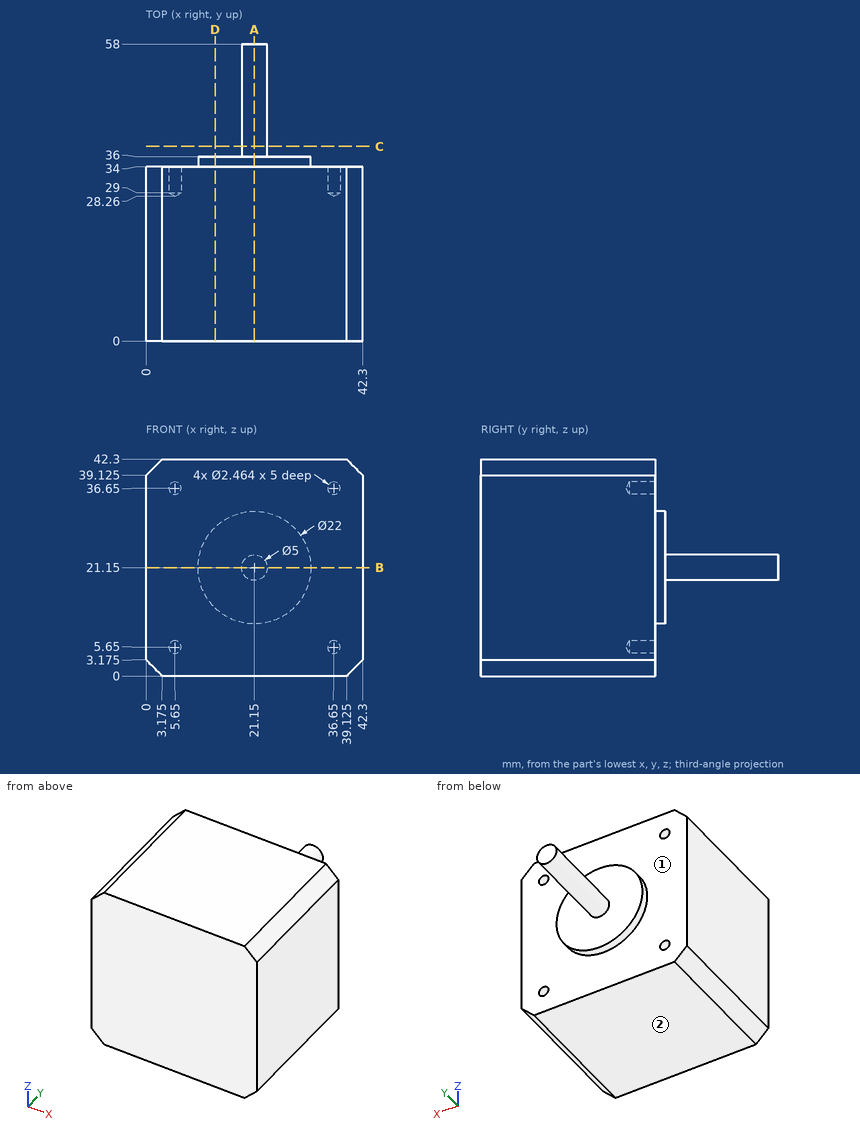
Could you check a few things on this drawing? It's one solid part, dimensions in mm from its lowest x, y, z. A direction names the side the tool comes from. Coordinates: 2 decimals unless noted, no trailing zeros. Write each loop counter-clockwise with the first axis right and the second up, starting at its lowest first coordinate (ties: lowest second). Pieces come first, ordered by that corner, then holes. Notation, with made-up numbers: (-36, 79.25) - (3, 79.25) arc R15 cw to (3, 88.25) - close; hole circle Ø1 at (-20, 14.25). An arc over 180 degrees is marked (long way). Write item = value, one per line.
1) Will these pins go through, and if not, where does the flat tip stop? pin 1 Ø4 at (x, z) = (36.65, 36.65) entering from +Y; pin 2 Ø1.5 at (x, z) = (5.65, 5.65) entering from +Y; pin 3 Ø5 at (x, y) = (23.5, 44.5) entering from +Z.
Result set:
pin_1 = 34
pin_2 = 28.71
pin_3 = 23.65
2) Suppose I cut it at A-A on x = 21.15. Please give me the cut outline in (y, z), plus the area to 3 significant figures.
Result set:
outline = (0, 0) - (34, 0) - (34, 10.15) - (36, 10.15) - (36, 18.65) - (58, 18.65) - (58, 23.65) - (36, 23.65) - (36, 32.15) - (34, 32.15) - (34, 42.3) - (0, 42.3) - close
area = 1,590 mm2
3) Suppose I cut it at D-D on x = 13.5. Please give me the cut outline in (y, z), plus the area to 3 significant figures.
Result set:
outline = (0, 0) - (34, 0) - (34, 13.25) - (36, 13.25) - (36, 29.05) - (34, 29.05) - (34, 42.3) - (0, 42.3) - close
area = 1,470 mm2
4) For the marked faces 1 and 2, which set-ups out of +Z, -Z, +X, -X, +Y, -Y let a thin tool reach every point of the face, with its end or its side?
Result set:
face_1 = +Y
face_2 = -Z, +X, -X, +Y, -Y
5) Suppose I cut it at C-C on y = 38. Please give me the cut outline in (x, z), plus the area to 3 significant figures.
Result set:
outline = circle Ø5 at (21.15, 21.15)
area = 19.6 mm2
6) Please list where these lines run through material, in increasing order: line 1 (Z direction, x = 5.65, y = 31.9); line 2 (Z direction, x = 5, y = 32). Write a range as [from, to].
Result set:
line_1 = [0, 4.42], [6.88, 35.42], [37.88, 42.3]
line_2 = [0, 4.6], [6.7, 35.6], [37.7, 42.3]
7) Suppose I cut it at B-B on z = 21.15. Please give me the cut outline in (x, y), plus the area to 3 significant figures.
Result set:
outline = (0, 0) - (42.3, 0) - (42.3, 34) - (32.15, 34) - (32.15, 36) - (23.65, 36) - (23.65, 58) - (18.65, 58) - (18.65, 36) - (10.15, 36) - (10.15, 34) - (0, 34) - close
area = 1,590 mm2
